```python
from build123d import *

# Parameters (mm, degrees)
F1_DEPTH = 76.2


# Not quite as in the source:
# - a feature of the source that left no trace in its solid (it failed there, or was rolled back) is left out


with BuildPart() as f1:
    # F0 (on Top) → F1 (new body)
    with BuildSketch(Plane.XY):
        with BuildLine():
            Line((0, 203.2), (0, 0))
            Line((0, 0), (63.5, 0))
            ThreePointArc((63.5, 0), (50.6075315628, 104.7268828907), (12.7, 203.2))
            Line((12.7, 203.2), (0, 203.2))
        make_face()
        with BuildLine():
            Line((-63.5, 0), (0, 0))
            Line((0, 0), (0, 203.2))
            Line((0, 203.2), (-12.7, 203.2))
            ThreePointArc((-12.7, 203.2), (-50.6075315628, 104.7268828907), (-63.5, 0))
        make_face()
        with BuildLine():
            Line((0, 215.9), (0, 203.2))
            Line((0, 203.2), (12.7, 203.2))
            ThreePointArc((12.7, 203.2), (8.9802561211, 212.1802561211), (0, 215.9))
        make_face()
        with BuildLine():
            Line((-12.7, 203.2), (0, 203.2))
            Line((0, 203.2), (0, 215.9))
            ThreePointArc((0, 215.9), (-8.9802561211, 212.1802561211), (-12.7, 203.2))
        make_face()
        with BuildLine():
            Line((0, -127), (0, 0))
            Line((0, 0), (-63.5, 0))
            Line((-63.5, 0), (-63.5, -101.6))
            ThreePointArc((-63.5, -101.6), (-60.1480633142, -115.7990316571), (-50.8, -127))
            Line((-50.8, -127), (0, -127))
        make_face()
        with BuildLine():
            Line((63.5, 0), (0, 0))
            Line((0, 0), (0, -127))
            Line((0, -127), (50.8, -127))
            ThreePointArc((50.8, -127), (60.1480633142, -115.7990316571), (63.5, -101.6))
            Line((63.5, -101.6), (63.5, 0))
        make_face()
    extrude(amount=F1_DEPTH)


solid = f1.part
```
The listing builds one solid part. Answer for the finished solid, in the listing's coordinates (mm). Coordinates: 2 decimals unless noted, no trailing zeros. Loops run counter-clockwise (first coordinate to the right, second up) from the corner with the lowest first, then second, coordinate; pieces in that order, holes last. Notation, with made-up numbers: M 57,74 L 114,74 A20 cw 114,94 Z; hole C 16.5,-10 d9. An arc over 180 degrees is marked long. Answer as a JSON object with one key per item and string values. Group by question number.
Item 1: Consider L1, parallel to Y at x = 0.5, z = 58; L2, parallel to X at y = 21.5, z = 61.5; L3, parallel to X at y = 178.5, z = 5.5. Determine where each line is inside the solid, lowest interval first.
Item 2: Section B-B (y = 124.5) is taken. Write down the section's boundary in (x, z), and give its area (3 significant figures).
Item 3: Section A-A (z = 63) is taken. Write down the section's boundary in (x, y), and give its area (3 significant figures).
Item 4: Each of these flat-tipped pins is pushed along its axis until it touches: P1, Ø4, axis at y = 127, z = 35.5, coming from the -X side; P2, Ø12, axis at x = -12, z = 65, coming from the +Y side. Where does it stop, or does it pass through?
Item 5: Section C-C (x = -43) is taken. Write down the section's boundary in (y, z), and give its area (3 significant figures).
Solved:
{
 "1": {"L1": "y = -127 to 215.89", "L2": "x = -62.96 to 62.96", "L3": "x = -24.88 to 24.88"},
 "2": {"outline": "M -45.16,0 L 45.16,0 L 45.16,76.2 L -45.16,76.2 Z", "area": "6,880 mm2"},
 "3": {"outline": "M -63.5,-101.6 A31.75 ccw -50.8,-127 L 50.8,-127 A31.75 ccw 63.5,-101.6 L 63.5,0 A431.8 ccw 12.7,203.2 A12.7 ccw -12.7,203.2 A431.8 ccw -63.5,0 Z", "area": "35,300 mm2"},
 "4": {"P1": "stops at x = -45.01", "P2": "stops at y = 214.39"},
 "5": {"outline": "M -127,0 L 131.47,0 L 131.47,76.2 L -127,76.2 Z", "area": "19,700 mm2"}
}
